Autodesk Inventor part; units mm, degrees
ref_plane "YZ Plane" through (0, 0, 0) normal (1, 0, 0) x (0, 1, 0)
ref_plane "XZ Plane" through (0, 0, 0) normal (0, 1, 0) x (-1, 0, 0)
ref_plane "XY Plane" through (0, 0, 0) normal (0, 0, 1) x (1, 0, 0)
sketch "Boceto1" plane through (0, 0, 0) normal (1, 0, 0) x (0, 1, 0)
  line L0 (0, 0) -> (-52.0696, 0)
  line L1 (-52.0696, 0) -> (-52.0696, 40)
  line L2 (-52.0696, 40) -> (0, 40)
  line L3 (0, 40) -> (0, 0)
  line L4 (0, 0) -> (51.9461, 0)
  line L5 (51.9461, 0) -> (51.9461, 40)
  line L6 (51.9461, 40) -> (0, 40)
  line L7 (0, 40) -> (0, 0)
  line L8 (-52.0696, 43) -> (-52.0696, 40) construction
  line L9 (51.9461, 43) -> (51.9461, 40) construction
  line L10 (36.9461, 40) -> (16.9461, 40)
  line L11 (16.9461, 40) -> (16.9461, 43)
  line L12 (16.9461, 43) -> (36.9461, 43)
  line L13 (36.9461, 43) -> (36.9461, 40)
  line L14 (-17.0696, 40) -> (-37.0696, 40)
  line L15 (-37.0696, 40) -> (-37.0696, 43)
  line L16 (-37.0696, 43) -> (-17.0696, 43)
  line L17 (-17.0696, 43) -> (-17.0696, 40)
  point P0 (16.9461, 40)
  dimension "d15" = 40
  dimension "d16" = 20
  dimension "d17" = 3
  dimension "d18" = 15
  dimension "d19" = 3
  dimension "d20" = 20
  dimension "d21" = 15
extrude "Extrusión1" add sketch "Boceto1" along normal blind 3
sketch "Boceto4" plane through (0, 0, 0) normal (-1, 0, 0) x (0, 0, 1)
  circle A0 centre (25, -37.0696) radius 1.6 construction
  circle A1 centre (25, -47.0696) radius 1.6 construction
  circle A2 centre (25, 36.9461) radius 1.6 construction
  circle A3 centre (25, 46.9461) radius 1.6 construction
  point P0 (0, 0)
hole "Agujero2" at (0, -47.0696, 25) at (0, -37.0696, 25) at (0, 36.9461, 25) at (0, 46.9461, 25) direction (1, 0, 0) diameter 3 end through all
sketch "Boceto5" plane through (3, 0, 0) normal (1, 0, 0) x (0, 0, -1)
  circle A0 centre (-23, 9.9416) radius 1.45 construction
  point P0 (0, 0)
hole "Agujero3" [suppressed]
sketch "ReferenciaEje" plane through (3, 0, 0) normal (1, 0, 0) x (0, 0, -1)
  circle A0 centre (-23, 9.9385) radius 1.65 construction
  line L0 (-40, 16.9461) -> (-40, -17.0696) construction
  line L1 (0, 51.9461) -> (-40, 51.9461) construction
  circle A1 centre (-21, 9.9385) radius 0.5
  point P0 (0, 0)
  dimension "d59" = 19
  dimension "d60" = 42.0076
  dimension "d61" = 1
sketch "Boceto9" plane through (3, 0, 0) normal (1, 0, 0) x (0, 0, -1)
  circle A0 centre (-15.9, 24.6885) radius 2.25 construction
  circle A1 centre (-26.1, 24.6885) radius 2.25 construction
  circle A2 centre (-15.9, -24.8115) radius 2.25 construction
  circle A3 centre (-26.1, -24.8115) radius 2.25 construction
  point P0 (0, 0)
hole "Agujero4" at (3, 24.6885, 15.9) at (3, 24.6885, 26.1) at (3, -24.8115, 26.1) at (3, -24.8115, 15.9) direction (-1, 0, 0) diameter 3 end through all
sketch "Boceto10" plane through (3, 0, 0) normal (1, 0, 0) x (0, 0, -1)
  line L0 (-11, 19.4385) -> (-11, -19.5615) construction
  line L1 (-30.5, 19.9385) -> (-11.5, 19.9385) construction
  line L2 (-31, -19.6129) -> (-31, 19.4898) construction
  line L3 (-11.4533, -20.0615) -> (-30.5467, -20.0615) construction
  line L4 (-10.8, 20.9385) -> (-31.2, 20.9385)
  line L5 (-31.2, 20.9385) -> (-31.2, -20.2615)
  line L6 (-31.2, -20.2615) -> (-10.8, -20.2615)
  line L7 (-10.8, -20.2615) -> (-10.8, 20.9385)
  point P0 (0, 0)
  point P1 (-11, -0.0615)
  dimension "d53" = 0.2
  dimension "d54" = 0.2
  dimension "d55" = 0.2
  dimension "d56" = 1
extrude "Extrusión4" cut sketch "Boceto10" against normal through all
fillet "Empalme1" radius 2 8 edges at (1.5, 51.9461, 0) (1.5, -52.0696, 0) (1.5, -52.0696, 40) (1.5, -37.0696, 43) (1.5, -17.0696, 43) (1.5, 16.9461, 43) (1.5, 36.9461, 43) (1.5, 51.9461, 40)
properties part number "ParedEnsambleMotor"
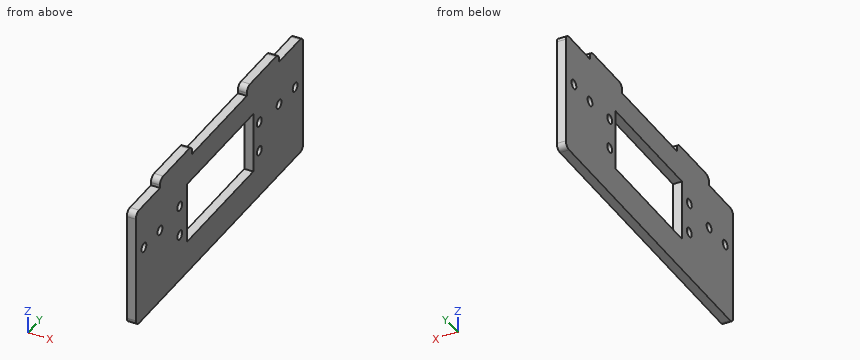
Input: part model. Units: mm. Frame: model coordinates. Round coordinates to 2 decimals unless told otherwise and drop trailing zeros. Loops run counter-clockwise (first coordinate to the right, second up) from the corner with the lowest first, then second, coordinate; pieces in that order, holes last. Notation, with made-up numbers: (65.25, 46.5) - (91.25, 46.5) arc R32 ccw to (91.25, 81.5) - close; hole circle Ø3 at (31, 3.5). An arc over 180 degrees is marked (long way). One line per item, written item: value. Start each with the question number.
(1) Section C-C, the plane x = 1.6. Count the separate pieces of the cut face and the enclosed holes in it, plus the area to 3 significant figures.
(2) Section A-A, the plane y = -1. Return loops of the section in (x, z).
(3) Contact query for flat-ended pins moving along their axis: P1, Ø1.5, axis at x = 0.5, y = 12, coming from the +Z side; P2, Ø0.5, axis at x = 1, z = 40.5, coming from the -Y side. Output: stop coordinate, or through.
(4) Ray query, line 1 (Y direction, x = 1.65, z = 15.9); line 2 (Z direction, x = 2.6, y = -1.5); line 3 (Y direction, x = 0.7, z = 21.5). Return the intervals inside material, ascending. Write a range as [from, to].
(5) Section B-B, the plane z = 15.9. Return loops of the section in (x, y).
Results below:
1. separate pieces: 1
1. enclosed holes: 9
1. area: 3,380 mm^2
2. outline: (0, 0) - (3, 0) - (3, 10.8) - (0, 10.8) - close; (0, 31.2) - (3, 31.2) - (3, 40) - (0, 40) - close
3. P1: z = 40
3. P2: y = -37.07
4. line 1: [-52.07, -26.31], [-23.31, -20.26], [20.94, 23.19], [26.19, 51.95]
4. line 2: [0, 10.8], [31.2, 40]
4. line 3: [-52.07, -20.26], [20.94, 51.95]
5. outline: (0, -52.07) - (3, -52.07) - (3, -26.31) - (0, -26.31) - close; (0, -23.31) - (3, -23.31) - (3, -20.26) - (0, -20.26) - close; (0, 20.94) - (3, 20.94) - (3, 23.19) - (0, 23.19) - close; (0, 26.19) - (3, 26.19) - (3, 51.95) - (0, 51.95) - close
